The drawing under review shows one solid part. Ordinate dimensions are in mm from its lowest x, y, z. A direction names the side the tool comes from. Round coordinates to 2 decimals unless told otherwise and drop trailing zeros. Write each loop counter-clockwise with the first axis right and the second up, starting at its lowest first coordinate (ties: lowest second). Pieces come first, ordered by that corner, then holes. Notation, with made-up numbers: (63, 23.25) -> (111, 23.25) arc R5 ccw to (111, 29.25) -> close; hole circle Ø4 at (-16, -28.75). An arc over 180 degrees is marked (long way). Write item = value, one per line. Start each with the question number.
Item 1: Machinability: for the marked faces 1, 2 and 3, which of the approach directions +Z, -Z, +X, -X, +Y, -Y give a long, thin tool a straight path to every point of the face, cutting with its end or side? Answer none if there is none.
Item 2: Add section D-D, the plane y = 1.5. State the section outline as (x, z) points, then the cut area to 3 significant figures.
Item 3: Add section B-B, the plane z = 49.5. State the section outline as (x, y) points, then the cut area to 3 significant figures.
Item 4: For pin 1 Ø4.5 at (y, z) = (2.5, 21.5) entering from +X; pin 2 Ø1 at (y, z) = (2, 17.5) entering from -X; pin 3 Ø2.5 at (x, z) = (4, 37) entering from -Y, all flat-tipped, find the tip position at first contact; note any pin that passes through.
Item 5: Add section C-C, the plane z = 60. State how many separate pieces and enclosed holes the cut face has, then the cut area to 3 significant figures.
Item 6: To check wall thickness, follow L1, parallel to X at y = 8.85, z = 60; L2, parallel to X at y = 6, z = 38; L3, parallel to Z at x = 62, y = 5.5 (1 decimal). State the ranges of each line that lie inside material, in increasing order.
Item 7: Mouldability with a two-part tool opening along X and no side actions: class the marked faces 4 and 5 as released by +X, released by -X, zero draft, split by the parting line, or undercut.
Item 8: Add section A-A, the plane x = 59.5. State the section outline as (y, z) points.
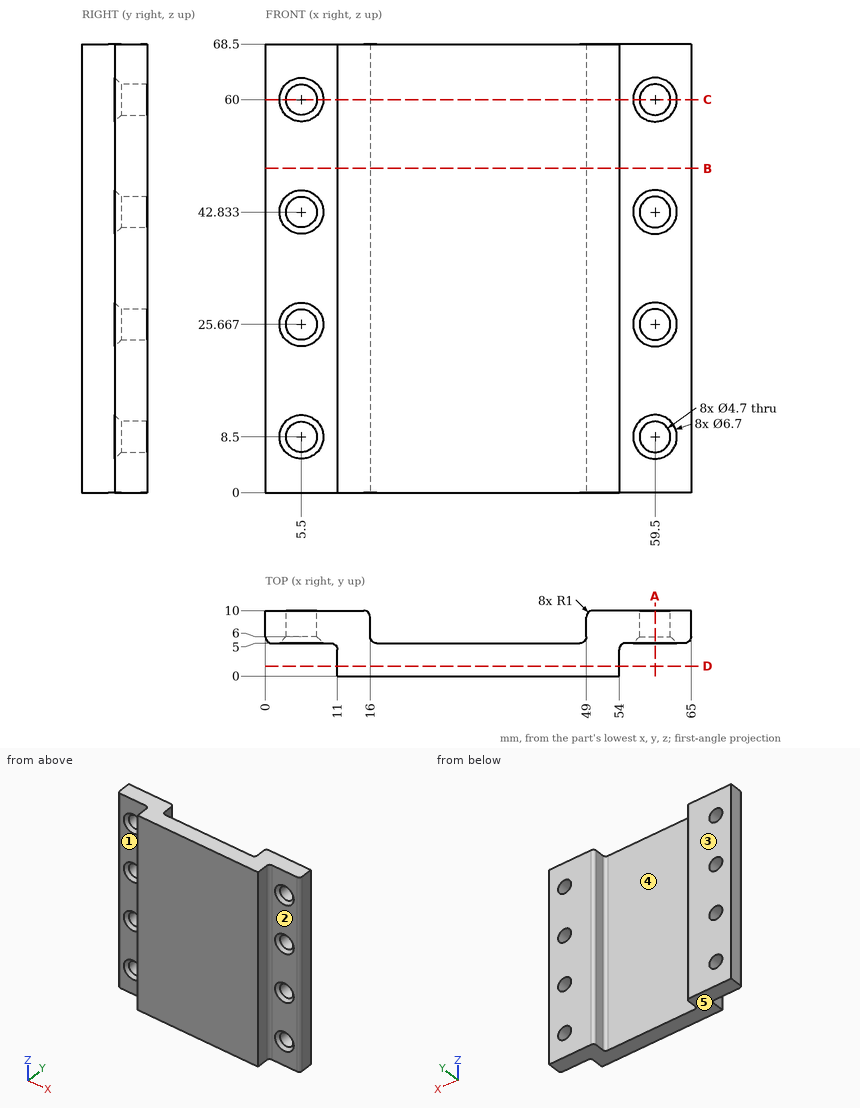
Result set:
q1.face_1 = +Z, -Z, -X, -Y
q1.face_2 = +Z, -Z, +X, -Y
q1.face_3 = +Z, -Z, +X, -X, +Y
q2.outline = (11, 0) -> (54, 0) -> (54, 68.5) -> (11, 68.5) -> close
q2.area = 2,950 mm²
q3.outline = (0, 6) arc R1 ccw to (1, 5) -> (10, 5) arc R1 cw to (11, 4) -> (11, 0) -> (54, 0) -> (54, 4) arc R1 cw to (55, 5) -> (64, 5) arc R1 ccw to (65, 6) -> (65, 10) -> (50, 10) arc R1 ccw to (49, 9) -> (49, 6) arc R1 cw to (48, 5) -> (17, 5) arc R1 cw to (16, 6) -> (16, 9) arc R1 ccw to (15, 10) -> (0, 10) -> close
q3.area = 375 mm²
q4.pin_1 = 54.34
q4.pin_2 = 11
q4.pin_3 = 5
q5.separate_pieces = 3
q5.enclosed_holes = 0
q5.area = 326 mm²
q6.L1 = 0 to 3.15, 7.85 to 16, 49 to 57.15, 61.85 to 65
q6.L2 = 0 to 16, 49 to 65
q6.L3 = 0 to 7.1, 9.9 to 24.3, 27 to 41.5, 44.2 to 58.6, 61.4 to 68.5
q7.face_4 = undercut
q7.face_5 = zero draft
q8.outline = (5, 0) -> (10, 0) -> (10, 6.15) -> (6, 6.15) -> (5, 5.15) -> close; (5, 11.85) -> (6, 10.85) -> (10, 10.85) -> (10, 23.32) -> (6, 23.32) -> (5, 22.32) -> close; (5, 29.02) -> (6, 28.02) -> (10, 28.02) -> (10, 40.48) -> (6, 40.48) -> (5, 39.48) -> close; (5, 46.18) -> (6, 45.18) -> (10, 45.18) -> (10, 57.65) -> (6, 57.65) -> (5, 56.65) -> close; (5, 63.35) -> (6, 62.35) -> (10, 62.35) -> (10, 68.5) -> (5, 68.5) -> close
